Here's how the part is built. I have some questions about the finished solid (model axes, mm). A direction names the side the tool comes from. Coordinates: 2 decimals unless noted, no trailing zeros. Loops run counter-clockwise (first coordinate to the right, second up) from the corner with the lowest first, then second, coordinate; pieces in that order, holes last. Notation, with made-up numbers: M 71.5,83.25 L 104.5,83.25 A20 ccw 104.5,93.25 Z; hole C -19,29 d1. An arc over 180 degrees is marked long. Use CSV: the item, a comma, the result in double quotes. Start each with the question number.
Q1. For pin 1 Ø3 at (x, z) = (50.5, 42) entering from -Y, with a flat end and sliding along its axis, tell me the tip position at first contact or that it passes through.
Q2. If we section it at A-A (x = 23.5): Please give me the cut outline in (y, z).
Q3. If we section it at D-D (z = 70.5): Please give me the cut outline in (x, y), and give its area (3 significant figures).
Q4. If we section it at C-C (x = 62.3): Please give me the cut outline in (y, z), and give its area (3 significant figures).
Q5. If we mould it in two halves opening along Z, with no side actions, what happens to faces 1 (the flat face through (19, -2, 29)), 2 (the flat face through (32, -2, 94)), 3 (the flat face through (46, -2, 61)), 4 (the flat face through (0, -2, 46))? For each: +Z half, -Z half, draft (parallel to the pull), parting line (faces both ways), or undercut.
Q6. If we section it at B-B (z = 91.5): Please give me the cut outline in (x, y).
Q7. Please list where these lines run through material, in increasing order: probe 1 along Z at (x, y) = (62.3, -2.15); probe 2 along Z at (x, y) = (23.5, -3.15); probe 3 along X at (y, z) = (-2.5, 85.5) (3 decimals). Write a range as [from, to].
Q8. Which directions (+Z, -Z, +X, -X, +Y, -Y) give clear straight access to the entire face, cutting with the end or side of a thin tool? Please do faces 5 (the flat face through (64.8, -2, 46)), 6 (the flat face through (36.725, -2, 59)).
from build123d import *

# Parameters (mm, degrees)
SKETCH_W        = 64.8
SKETCH_H        = 94
PAD_DEPTH       = 5
POCKET_DEPTH    = 1.2
SKETCH002_R     = 1
POCKET001_DEPTH = 3.801
SKETCH003_W     = 18.75
SKETCH003_H     = 4
POCKET002_DEPTH = 3.801
SKETCH004_R     = 2
POCKET003_DEPTH = 5.001


with BuildPart() as part:
    # Sketch → Pad (new body)
    with BuildSketch(Plane.XZ):
        with Locations((32.4, 47)):
            Rectangle(SKETCH_W, SKETCH_H)
    extrude(amount=PAD_DEPTH)

    # Sketch001 (on Face6 of Pad) → Pocket (cut)
    with BuildSketch(Plane.XZ.offset(5)):
        Polygon((5, 5), (32.4, 5), (59.8, 5), (59.8, 33), (59.8, 61), (59.8, 89), (32.4, 89), (5, 89), (5, 61), (5, 33), align=None)
    extrude(amount=-POCKET_DEPTH, mode=Mode.SUBTRACT)

    # Sketch002 (on Face17 of Pocket) → Pocket001 (cut, through all)
    with BuildSketch(Plane.XZ.offset(3.8)):
        with Locations((7, 87)):
            Circle(SKETCH002_R)
        with Locations((30.4, 87)):
            Circle(SKETCH002_R)
        with Locations((34.4, 87)):
            Circle(SKETCH002_R)
        with Locations((57.8, 87)):
            Circle(SKETCH002_R)
        with Locations((7, 63)):
            Circle(SKETCH002_R)
        with Locations((30.4, 63)):
            Circle(SKETCH002_R)
        with Locations((34.4, 63)):
            Circle(SKETCH002_R)
        with Locations((57.8, 63)):
            Circle(SKETCH002_R)
        with Locations((57.8, 59)):
            Circle(SKETCH002_R)
        with Locations((34.4, 59)):
            Circle(SKETCH002_R)
        with Locations((30.4, 59)):
            Circle(SKETCH002_R)
        with Locations((7, 59)):
            Circle(SKETCH002_R)
        with Locations((7, 35)):
            Circle(SKETCH002_R)
        with Locations((7, 31)):
            Circle(SKETCH002_R)
        with Locations((30.4, 31)):
            Circle(SKETCH002_R)
        with Locations((30.4, 35)):
            Circle(SKETCH002_R)
        with Locations((34.4, 35)):
            Circle(SKETCH002_R)
        with Locations((34.4, 31)):
            Circle(SKETCH002_R)
        with Locations((57.8, 31)):
            Circle(SKETCH002_R)
        with Locations((57.8, 35)):
            Circle(SKETCH002_R)
        with Locations((7, 7)):
            Circle(SKETCH002_R)
        with Locations((30.4, 7)):
            Circle(SKETCH002_R)
        with Locations((34.4, 7)):
            Circle(SKETCH002_R)
        with Locations((57.8, 7)):
            Circle(SKETCH002_R)
    extrude(amount=-POCKET001_DEPTH, mode=Mode.SUBTRACT)

    # Sketch003 (on Face41 of Pocket001) → Pocket002 (cut, through all)
    with BuildSketch(Plane.XZ.offset(3.8)):
        with Locations((18.7, 31)):
            Rectangle(SKETCH003_W, SKETCH003_H)
        with Locations((46.1, 31)):
            Rectangle(SKETCH003_W, SKETCH003_H)
        with Locations((18.7, 59)):
            Rectangle(SKETCH003_W, SKETCH003_H)
        with Locations((46.1, 59)):
            Rectangle(SKETCH003_W, SKETCH003_H)
        with Locations((18.7, 87)):
            Rectangle(SKETCH003_W, SKETCH003_H)
        with Locations((46.1, 87)):
            Rectangle(SKETCH003_W, SKETCH003_H)
    extrude(amount=-POCKET002_DEPTH, mode=Mode.SUBTRACT)

    # Sketch004 (on Face5 of Pocket002) → Pocket003 (cut, through all)
    with BuildSketch(Plane.XZ.offset(5)):
        with Locations((2.5, 2.5)):
            Circle(SKETCH004_R)
        with Locations((62.3, 2.5)):
            Circle(SKETCH004_R)
        with Locations((2.5, 91.5)):
            Circle(SKETCH004_R)
        with Locations((62.3, 91.5)):
            Circle(SKETCH004_R)
    extrude(amount=-POCKET003_DEPTH, mode=Mode.SUBTRACT)


solid = part.part
Results below:
1,pin 1,"y = -3.8"
2,outline,"M -5,0 L 0,0 L 0,29 L -3.8,29 L -3.8,5 L -5,5 Z; M -5,89 L 0,89 L 0,94 L -5,94 Z; M -3.8,33 L 0,33 L 0,57 L -3.8,57 Z; M -3.8,61 L 0,61 L 0,85 L -3.8,85 Z"
3,outline,"M 0,-5 L 5,-5 L 5,-3.8 L 59.8,-3.8 L 59.8,-5 L 64.8,-5 L 64.8,0 L 0,0 Z"
3,area,"258 mm^2"
4,outline,"M -5,0 L 0,0 L 0,0.5 L -5,0.5 Z; M -5,4.5 L 0,4.5 L 0,89.5 L -5,89.5 Z; M -5,93.5 L 0,93.5 L 0,94 L -5,94 Z"
4,area,"430 mm^2"
5,face 1,"undercut"
5,face 2,"+Z half"
5,face 3,"undercut"
5,face 4,"draft"
6,outline,"M 0,-5 L 0.5,-5 L 0.5,0 L 0,0 Z; M 4.5,-5 L 60.3,-5 L 60.3,0 L 4.5,0 Z; M 64.3,-5 L 64.8,-5 L 64.8,0 L 64.3,0 Z"
7,probe 1,"[0, 0.5], [4.5, 89.5], [93.5, 94]"
7,probe 2,"[0, 29], [33, 57], [61, 85], [89, 94]"
7,probe 3,"[0, 9.325], [28.075, 36.725], [55.475, 64.8]"
8,face 5,"+Z, -Z, +X, +Y, -Y"
8,face 6,"+Y, -Y"
